Verification items for this drawing (mm, ordinates from the low corner). Give positions to 0.01 mm unless a question says otherwise; leave off trailing zeros. Loops run counter-clockwise (first coordinate to the right, second up) from the corner with the lowest first, then second, coordinate; pieces in that order, holes last. Notation, with made-up numbers: (19.25, -38.75) - (31.25, -38.75) arc R15 ccw to (31.25, -18.75) - close; hole circle Ø2 at (3, -38). An arc over 180 degrees is marked (long way). One line per question, with ' | ' between items. Start each with the question number.
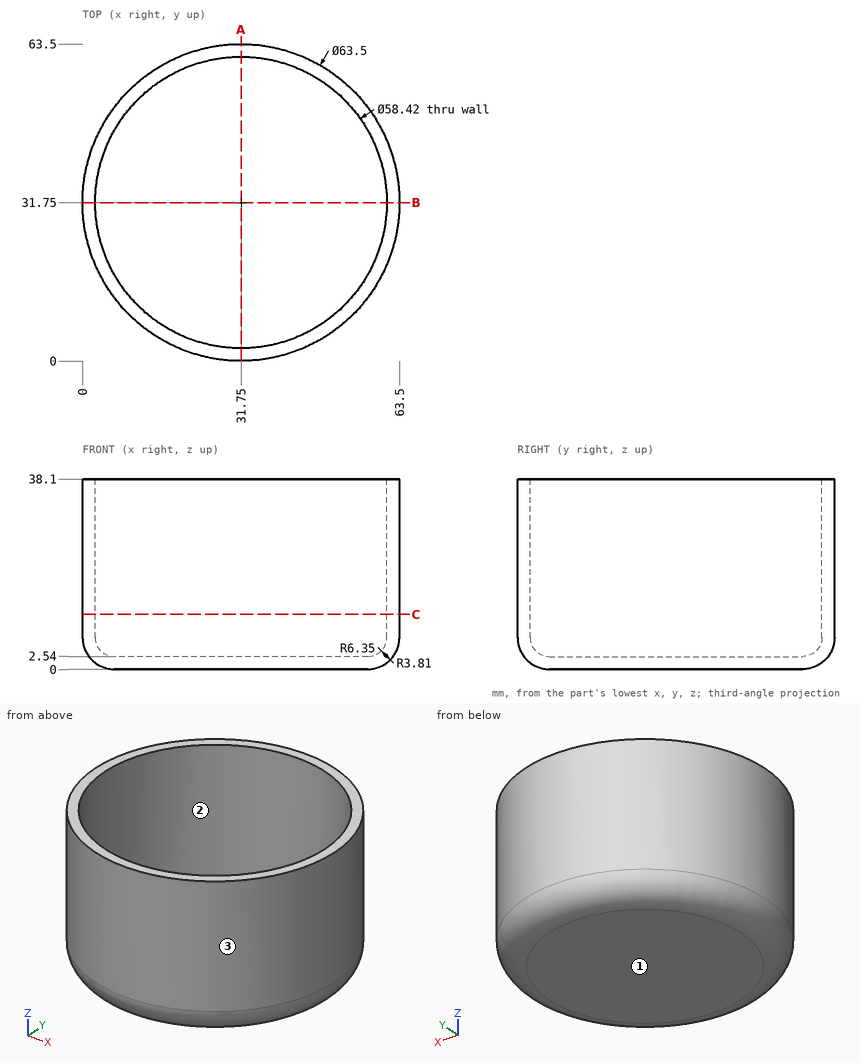
(1) Material ranges on line 1 (Y direction, x = 31.75, z = 13); line 2 (X direction, y = 31, z = 14); line 3 (Z direction, x = 37, y = 11.5), recorded low to high.
(2) Mould release check, pull along X, two halves, no side actions. Record for the marked faces 1, 2 and 3: pulls with the +X half, pulls with the -X half, needs draft (parallel to the pull), parting line crosses it, or undercut.
(3) Section check A-A, the plane x = 31.75. Record the boundary of the cut face in (y, z).
(4) Depth check by flat-ended pin: pin 1 Ø4 at (y, z) = (13.5, 12) entering from +X; pin 2 Ø1.5 at (y, z) = (10.5, 5.5) entering from +X; pin 3 Ø1 at (x, z) = (33.5, 31.5) entering from +Y; pin 4 Ø12 at (y, z) = (31, 9) entering from +X. Enter the tip coordinate at first touch or a pass-through.
(5) Section check C-C, the plane z = 11. Record the boundary of the cut face in (x, y), and give its area (3 significant figures).
Numbers:
1) line 1: 0 to 2.54, 60.96 to 63.5 | line 2: 0.01 to 2.55, 60.95 to 63.49 | line 3: 0 to 2.54
2) face 1: needs draft | face 2: undercut | face 3: parting line crosses it
3) outline: (0, 6.35) arc R6.35 ccw to (6.35, 0) - (57.15, 0) arc R6.35 ccw to (63.5, 6.35) - (63.5, 38.1) - (60.96, 38.1) - (60.96, 6.35) arc R3.81 cw to (57.15, 2.54) - (6.35, 2.54) arc R3.81 cw to (2.54, 6.35) - (2.54, 38.1) - (0, 38.1) - close
4) pin 1: x = 59.03 | pin 2: x = 55.93 | pin 3: y = 63.48 | pin 4: x = 63.5
5) outline: circle Ø63.5 at (31.75, 31.75); hole circle Ø58.42 at (31.75, 31.75) | area: 486 mm^2
